```python
from build123d import *

# Parameters (mm, degrees)
SKETCH1_R           = 12.121929558
BOSS_EXTRUDE1_DEPTH = 70
SKETCH2_R           = 6.435362547
CUT_EXTRUDE1_DEPTH  = 60
CHAMFER1_SIZE       = 4
CHAMFER1_SIZE2      = 45.720209211


with BuildPart() as part:
    # Sketch1 → Boss-Extrude1 (new body)
    with BuildSketch(Plane.XY):
        Circle(SKETCH1_R)
    extrude(amount=BOSS_EXTRUDE1_DEPTH)

    # Sketch2 → Cut-Extrude1 (cut)
    with BuildSketch(Plane.XY.offset(70)):
        Circle(SKETCH2_R)
    extrude(amount=-CUT_EXTRUDE1_DEPTH, mode=Mode.SUBTRACT)

    # Chamfer1
    chamfer1_edges = [part.edges().sort_by_distance(p)[0] for p in [
        (-6.435362547, 0, 70),
    ]]
    chamfer1_side = [part.faces().sort_by_distance(p)[0] for p in [
        (-11.779069614, 0, 70),
    ]]
    chamfer(chamfer1_edges, length=CHAMFER1_SIZE, length2=CHAMFER1_SIZE2, reference=chamfer1_side[0])


solid = part.part
```
CAD build for the part. Positions are in the model's coordinates, mm. A direction names the side the tool comes from. Give positions to 0.01 mm unless a question says otherwise; leave off trailing zeros. Order: outer loops, then holes, each group sorted by start corner. A loop starts at its lowest first (then second) coordinate and runs counter-clockwise, first axis right, second up. Notation, with made-up numbers: M -29.5,-21 L 16.5,-21 A17 cw 16.5,10 Z; hole C -20,60.25 d8. An arc over 180 degrees is marked long. Put each result on its own line as item: value. Start each with the question number.
(1) Saw through at D-D, the plane z = 63.5. Write the cut outline in (x, y), then the cut area to 3 significant figures.
(2) Flat gauge pins, fed straight in: pin 1 Ø1 at (y, z) = (9, 49.5) entering from -X; pin 2 Ø14 at (x, y) = (3, 2) entering from +Z; pin 3 Ø1.5 at (x, z) = (-4, 40) entering from -Y; pin 4 Ø6 at (y, z) = (-6.5, 57.5) entering from -X. Where does each tip first touch, or does it go through?
(3) Saw through at B-B, the plane y = 0. Write the cut outline in (x, z), then the cut area to 3 significant figures.
(4) Saw through at A-A, the plane z = 17. Write the cut outline in (x, y), then the cut area to 3 significant figures.
(5) Drill centre lines: line 1 along Y through (x, z) = (0, 16.75); line 2 along Z through (x, y) = (2.75, 2.5); line 3 along X through (y, z) = (-5, 16). Where is each one in solid material? Low to high.
(6) Mould opens along Y. For faces 1 (the flat face through (0, 0, 10)), 2 (the cylindrical face through (-9.6, -7.4, 34.5)), 3 (the flat face through (4, 10, 70)) say: +Y half, -Y half, draft (parallel to the pull), parting line (faces both ways), or undercut.
(7) Which spindle directions (+Z, -Z, +X, -X, +Y, -Y) get a long thin tool onto all of the face, cutting with end or side? Do faces 4 (the flat face through (0, 0, 0)), 5 (the cylindrical face through (-0.84, 6.38, 17.24)). Say none if no direction does.
Check result:
1. outline: C 0,0 d24.24; hole C 0,0 d19.73
1. area: 156 mm2
2. pin 1: stops at x = -8.64
2. pin 2: stops at z = 70
2. pin 3: stops at y = -11.68
2. pin 4: stops at x = -11.61
3. outline: M -12.12,0 L 12.12,0 L 12.12,70 L 10.44,70 L 6.44,24.28 L 6.44,10 L -6.44,10 L -6.44,24.28 L -10.44,70 L -12.12,70 Z
3. area: 742 mm2
4. outline: C 0,0 d24.24; hole C 0,0 d12.87
4. area: 332 mm2
5. line 1: y = -12.12 to -6.44, 6.44 to 12.12
5. line 2: z = 0 to 10
5. line 3: x = -11.04 to -4.05, 4.05 to 11.04
6. face 1: undercut
6. face 2: parting line
6. face 3: draft
7. face 4: -Z, +X, -X, +Y, -Y
7. face 5: +Z
